The listing builds one solid part. Answer for the finished solid, in the listing's coordinates (mm). Face numbers are marked on the shaded views. A direction names the side the tool comes from. Coordinates: 2 decimals unless noted, no trailing zeros. Order: outer loops, then holes, each group sorted by start corner. A loop starts at its lowest first (then second) coordinate and runs counter-clockwise, first axis right, second up. Notation, with made-up numbers: (53, -14.75) - (110, -14.75) arc R36 ccw to (110, 21.25) - close; hole circle Ø6 at (-34, 80). An arc over 180 degrees is marked (long way). Use one line per item in the form item = value. Start each with the question number.
Item 1: Section D-D, the plane x = 238 is taken. Write down the section's boundary in (y, z), and give its area (3 significant figures).
Item 2: Section A-A, the plane y = 57 is taken. Write down the section's boundary in (x, z).
Item 3: Section C-C, the plane z = 64 is taken. Write down the section's boundary in (x, y), and give its area (3 significant figures).
Item 4: A tool of negligible diameter and unlimited length cuts with its end or side. For the marked faces 4, 5 and 6, from which of +Z, -Z, +X, -X, +Y, -Y can it reach the whole face along a straight path? Write none if from no direction.
Item 5: Section B-B, the plane x = 38 is taken. Write down the section's boundary in (y, z).
Item 6: The mould has two halves that part along Y. Classify the marked faces 1, 2 and 3: released by +Y, released by -Y, zero draft, split by the parting line, or undercut.
Item 7: Consider line 1 along Z through (x, y) = (398, 93.5); line 2 along X through (y, z) = (56.5, 89.5); line 3 along Y through (x, z) = (435, 61). Determine where each line is inside the solid, lowest interval first. Write a range as [from, to].
Item 8: Each of these flat-tipped pins is pushed along its axis until it touches: pin 1 Ø12 at (x, z) = (232.5, 40.5) entering from -Y; pin 2 Ø9 at (x, y) = (253.5, 258) entering from +Z; pin 3 Ø2 at (y, z) = (214, 86) entering from +X. Where does it stop, or does it pass through?
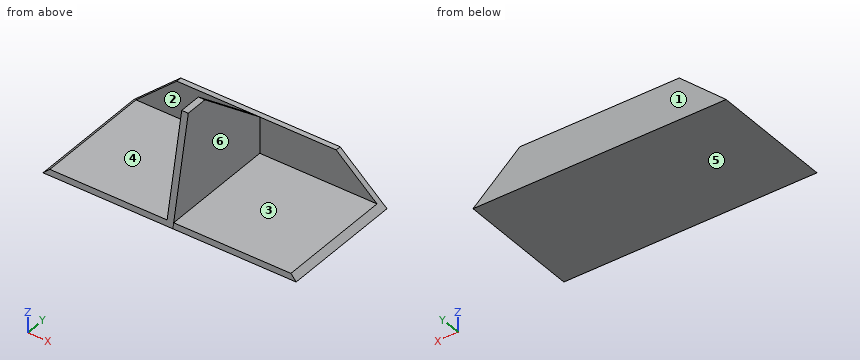
from build123d import *

# Parameters (mm, degrees)
SKETCH_1_W          = 540
SKETCH_1_H          = 265
EXTRUDE_505_DEPTH   = 11.5
SKETCH_2_W          = 540
SKETCH_2_H          = 11.5
EXTRUDE_1_DEPTH     = 77.5
CUT_EXTRUDE_1_DEPTH = 609.067430471
SKETCH_5_W          = 14
SKETCH_5_H          = 253.5
EXTRUDE_2_DEPTH     = 208.5
CUT_EXTRUDE_3_DEPTH = 442.988687638
CUT_EXTRUDE_4_DEPTH = 442.988687638


with BuildPart() as part:
    # 草图1 → Extrude 505 (new body)
    with BuildSketch(Plane.XY):
        with Locations((270, 132.5)):
            Rectangle(SKETCH_1_W, SKETCH_1_H)
    extrude(amount=EXTRUDE_505_DEPTH)

    # 草图2 → 凸台-拉伸1 (add)
    with BuildSketch(Plane.XY.offset(11.5)):
        with Locations((270, 259.25)):
            Rectangle(SKETCH_2_W, SKETCH_2_H)
    extrude(amount=EXTRUDE_1_DEPTH)

    # 草图3 → 切除-拉伸1 (cut, through all)
    with BuildSketch(Plane(origin=(0, 265, 0), x_dir=(-1, 0, 0), z_dir=(0, 1, 0))):
        Polygon((0, 0), (-100, 89), (0, 89), align=None)
        Polygon((-540, 0), (-440, 89), (-540, 89), align=None)
    extrude(amount=-CUT_EXTRUDE_1_DEPTH, mode=Mode.SUBTRACT)

    # 草图5 → 凸台-拉伸2 (add)
    with BuildSketch(Plane.XY.offset(11.5)):
        with Locations((270, 126.75)):
            Rectangle(SKETCH_5_W, SKETCH_5_H)
    extrude(amount=EXTRUDE_2_DEPTH)

    # 草图6 → 切除-拉伸3 (cut, through all)
    with BuildSketch(Plane(origin=(277, 0, 0), x_dir=(0, 0, -1), z_dir=(1, 0, 0))):
        Polygon((-89, 253.5), (-220, 93.5), (-220, 253.5), align=None)
        Polygon((-220, 45), (0, 0), (-220, 0), align=None)
    extrude(amount=-CUT_EXTRUDE_3_DEPTH, mode=Mode.SUBTRACT)

    # 草图7 → 切除-拉伸4 (cut, through all)
    with BuildSketch(Plane.ZY.offset(-277)):
        Polygon((0, 0), (11.5, 2.352272727), (11.5, 0), align=None)
    extrude(amount=-CUT_EXTRUDE_4_DEPTH, mode=Mode.SUBTRACT)


solid = part.part
Response:
q1.outline = (0, 0) - (265, 0) - (265, 89) - (253.5, 89) - (253.5, 11.5) - (2.35, 11.5) - close
q1.area = 3,930 mm2
q2.outline = (0, 0) - (540, 0) - (527.08, 11.5) - (277, 11.5) - (277, 220) - (263, 220) - (263, 11.5) - (12.92, 11.5) - close
q3.outline = (71.91, 253.5) - (263, 253.5) - (263, 13.09) - (277, 13.09) - (277, 253.5) - (468.09, 253.5) - (468.09, 265) - (71.91, 265) - close
q3.area = 7,920 mm2
q4.face_4 = +Z, -X, -Y
q4.face_5 = -Z, +X, -X, +Y, -Y
q4.face_6 = +Z, +X, -Y
q5.outline = (0, 0) - (265, 0) - (265, 33.82) - (253.5, 33.82) - (253.5, 11.5) - (2.35, 11.5) - close
q6.face_1 = released by +Y
q6.face_2 = released by -Y
q6.face_3 = zero draft
q7.line_1 = [0, 11.5]
q7.line_2 = [263, 277]
q7.line_3 = [253.5, 265]
q8.pin_1 = 253.5
q8.pin_2 = 89
q8.pin_3 = 277
